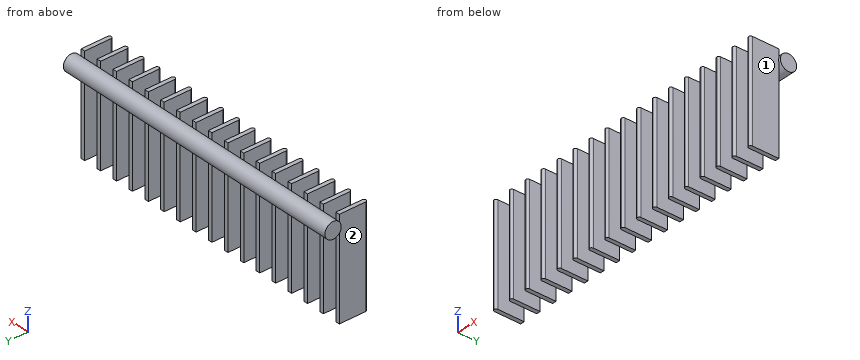
from build123d import *

# Parameters (mm, degrees)
F0_R          = 20
F1_DEPTH      = 375
F3_W          = 10
F3_H          = 70
F4_DEPTH      = 25
F4_DEPTH_BACK = 220
F5_R          = 4.99999
F6_R          = 4.99999


# Not quite as in the source:
# - a fillet or chamfer is up to 0.001 mm smaller than in the source, because OpenCascade refuses the exact size
# - a feature names something its author has since deleted; it is built from what else it names


with BuildPart() as f1:
    # F0 (on Right) → F1 (new body, symmetric)
    with BuildSketch(Plane.YZ):
        with Locations((-45, 220)):
            Circle(F0_R)
    extrude(amount=F1_DEPTH, both=True)

    # F3 (on plane+point) → F4 (join, two sides)
    with BuildSketch(Plane.XY.offset(220)) as f4_sk:
        with Locations((-365, -99.5)):
            Rectangle(F3_W, F3_H)
        with Locations((-319.375, -99.5)):
            Rectangle(F3_W, F3_H)
        with Locations((-273.75, -99.5)):
            Rectangle(F3_W, F3_H)
        with Locations((-228.125, -99.5)):
            Rectangle(F3_W, F3_H)
        with Locations((-182.5, -99.5)):
            Rectangle(F3_W, F3_H)
        with Locations((-136.875, -99.5)):
            Rectangle(F3_W, F3_H)
        with Locations((-91.25, -99.5)):
            Rectangle(F3_W, F3_H)
        with Locations((-45.625, -99.5)):
            Rectangle(F3_W, F3_H)
        with Locations((0, -99.5)):
            Rectangle(F3_W, F3_H)
        with Locations((45.625, -99.5)):
            Rectangle(F3_W, F3_H)
        with Locations((91.25, -99.5)):
            Rectangle(F3_W, F3_H)
        with Locations((136.875, -99.5)):
            Rectangle(F3_W, F3_H)
        with Locations((182.5, -99.5)):
            Rectangle(F3_W, F3_H)
        with Locations((228.125, -99.5)):
            Rectangle(F3_W, F3_H)
        with Locations((273.75, -99.5)):
            Rectangle(F3_W, F3_H)
        with Locations((319.375, -99.5)):
            Rectangle(F3_W, F3_H)
        with Locations((365, -99.5)):
            Rectangle(F3_W, F3_H)
    extrude(amount=F4_DEPTH)
    extrude(f4_sk.sketch, amount=-F4_DEPTH_BACK)

    # F5 (radius 5 in the source; OpenCascade refuses exactly that, so slightly less here)
    f5_edges = [f1.edges().sort_by_distance(p)[0] for p in [
        (-360, -134.5, 122.5),
        (-370, -134.5, 122.5),
    ]]
    fillet(f5_edges, radius=F5_R)

    # F6 (radius 5 in the source; OpenCascade refuses exactly that, so slightly less here)
    f6_edges = [f1.edges().sort_by_distance(p)[0] for p in [
        (-324.375, -134.5, 122.5),
        (-314.375, -134.5, 122.5),
        (-278.75, -134.5, 122.5),
        (-268.75, -134.5, 122.5),
        (-223.125, -134.5, 122.5),
        (-233.125, -134.5, 122.5),
        (-177.5, -134.5, 122.5),
        (-187.5, -134.5, 122.5),
        (-131.875, -134.5, 122.5),
        (-141.875, -134.5, 122.5),
        (-86.25, -134.5, 122.5),
        (-96.25, -134.5, 122.5),
        (-40.625, -134.5, 122.5),
        (-50.625, -134.5, 122.5),
        (5, -134.5, 122.5),
        (-5, -134.5, 122.5),
        (50.625, -134.5, 122.5),
        (40.625, -134.5, 122.5),
        (86.25, -134.5, 122.5),
        (96.25, -134.5, 122.5),
        (131.875, -134.5, 122.5),
        (141.875, -134.5, 122.5),
        (187.5, -134.5, 122.5),
        (177.5, -134.5, 122.5),
        (233.125, -134.5, 122.5),
        (223.125, -134.5, 122.5),
        (278.75, -134.5, 122.5),
        (268.75, -134.5, 122.5),
        (324.375, -134.5, 122.5),
        (314.375, -134.5, 122.5),
        (370, -134.5, 122.5),
        (360, -134.5, 122.5),
    ]]
    fillet(f6_edges, radius=F6_R)


solid = f1.part
The model under review builds one solid part; all positions refer to its coordinate system, in mm. Face numbers are marked on the shaded views. Give positions to 0.01 mm unless a question says otherwise; leave off trailing zeros. Write each loop counter-clockwise with the first axis right and the second up, starting at its lowest first coordinate (ties: lowest second). Pieces come first, ordered by that corner, then holes. Notation, with made-up numbers: M 53.5,19.25 L 59.5,19.25 A20 ccw 59.5,37.25 Z; hole C 69,56 d9. An arc over 180 degrees is marked long. One line per question, with ' | ' between items. Start each with the question number.
Item 1: Draft analysis for pull direction X (two halves, no side actions). For the marked faces 1 and 2, state which applies: released by +X, released by -X, zero draft, split by the parting line, or undercut.
Item 2: We need section C-C on x = 21. Write out the cut boundary in (y, z), plus the area to 3 significant figures.
Item 3: We need section A-A on z = 91. Give the number of separate pieces and of enclosed holes in the cut face, plus the area to 3 significant figures.
Item 4: We need section D-D on y = -45. Write out the cut boundary in (x, z).
Item 5: Wall thickness on line 1 (Y direction, x = 195.5, z = 220.5); line 2 (Z direction, x = 329.5, y = -42.5); line 3 (Y direction, x = -279, z = 234.5): over which ranges is each line inside the solid? List them lowest first. Write a range as from..to.
Item 6: For pin 1 (8 mm diameter, centred on x = -226, z = 113.5, fed in from +Y); pin 2 (3 mm diameter, centred on x = 271.5, z = 233.5, fed in from +Y); pin 3 (12 mm diameter, centred on y = -118.5, z = 103, fed in from +X), all flat-tipped, find the tip position at first contact; note any pin that passes through.
Results found:
1) face 1: released by +X | face 2: released by -X
2) outline: C -45,220 d40 | area: 1,260 mm2
3) separate pieces: 17 | enclosed holes: 0 | area: 11,700 mm2
4) outline: M -375,200 L 375,200 L 375,240 L -375,240 Z
5) line 1: y = -64.99..-25.01 | line 2: z = 200.16..239.84 | line 3: y = -58.77..-31.23
6) pin 1: stops at y = -64.5 | pin 2: stops at y = -29 | pin 3: stops at x = 370
